```python
from build123d import *

# Parameters (mm, degrees)
SKETCH_1_W      = 33
SKETCH_1_H      = 18
EXTRUDE_1_DEPTH = 1.5
EXTRUDE_2_DEPTH = 0.6
EXTRUDE_3_DEPTH = 2


with BuildPart() as part:
    # Эскиз1 → Бобышка-Вытянуть1 (new body)
    with BuildSketch(Plane.XY):
        with Locations((16.5, 9)):
            Rectangle(SKETCH_1_W, SKETCH_1_H)
    extrude(amount=EXTRUDE_1_DEPTH)

    # Эскиз2 → Бобышка-Вытянуть2 (add)
    with BuildSketch(Plane.XY.offset(1.5)):
        Polygon((18, 12.535533906), (21.535533906, 9), (18, 5.464466094), (14.464466094, 9), align=None)
    extrude(amount=EXTRUDE_2_DEPTH)

    # Эскиз3 → Бобышка-Вытянуть3 (add)
    with BuildSketch(Plane.XY.offset(1.5)):
        with BuildLine():
            Line((6.886292912, 6), (6.886292912, 12))
            ThreePointArc((6.886292912, 12), (8.886292912, 14), (10.886292912, 12))
            Line((10.886292912, 12), (10.886292912, 6))
            ThreePointArc((10.886292912, 6), (8.886292912, 4), (6.886292912, 6))
        make_face()
    extrude(amount=EXTRUDE_3_DEPTH)


solid = part.part
```
For this review, take the finished solid that the model builds, in its own axes (mm). A direction names the side the tool comes from. Round coordinates to 2 decimals unless told otherwise and drop trailing zeros. Write each loop counter-clockwise with the first axis right and the second up, starting at its lowest first coordinate (ties: lowest second). Pieces come first, ordered by that corner, then holes. Notation, with made-up numbers: (-13, 70) - (16, 70) arc R24 ccw to (16, 98) - close; hole circle Ø7 at (23.5, 74). An arc over 180 degrees is marked (long way). Use CSV: the item, a comma, the result in double quotes.
1) Add section B-B on y = 10. Write out the cut boundary in (x, z).
Conclusion:
outline,"(0, 0) - (33, 0) - (33, 1.5) - (20.54, 1.5) - (20.54, 2.1) - (15.46, 2.1) - (15.46, 1.5) - (10.89, 1.5) - (10.89, 3.5) - (6.89, 3.5) - (6.89, 1.5) - (0, 1.5) - close"
2) For faces 1 (the flat face through (19.793, 7.257, 1.796)), 2 (the flat face through (16, 7, 1.5)), 3 (the flat face through (19.743, 10.793, 1.796)), list the 3-axis set-ups (+Z, -Z, +X, -X, +Y, -Y) from which the entire face can be reached by the end or side of a thin tool; tool diameter is ignored.
Conclusion:
face 1,"+Z, +X, -Y"
face 2,"+Z"
face 3,"+Z, +X, +Y"
3) Add section C-C on z = 2.75. Write out the cut boundary in (x, y).
Conclusion:
outline,"(6.89, 6) arc R2 ccw to (10.89, 6) - (10.89, 12) arc R2 ccw to (6.89, 12) - close"
4) Clearance check with flat-ended pins moving along their axes: pin 1 Ø1.5 at (x, z) = (7.5, 3) entering from +Y; pin 2 Ø1.5 at (x, z) = (3.5, 3) entering from +Y; pin 3 Ø1 at (x, y) = (28.5, 3.5) entering from +Z; pin 4 Ø2 at (x, y) = (16.5, 8) entering from +Z. State where each tip first meets the part, or that it passes through.
Conclusion:
pin 1,"stops at y = 13.9"
pin 2,"passes through"
pin 3,"stops at z = 1.5"
pin 4,"stops at z = 2.1"
5) Wall thickness on line 1 along Z through (x, y) = (4, 13); line 2 along X through (y, z) = (9.5, 2.35); line 3 along X through (y, z) = (6, 1.7): over which ranges is each line inside the solid? List them lowest first. Write a range as from..to.
Conclusion:
line 1,"z = 0..1.5"
line 2,"x = 6.89..10.89"
line 3,"x = 6.89..10.89, 17.46..18.54"
6) Add section A-A on x = 10. Write out the cut boundary in (y, z), and give its area (3 significant figures).
Conclusion:
outline,"(0, 0) - (18, 0) - (18, 1.5) - (13.66, 1.5) - (13.66, 3.5) - (4.34, 3.5) - (4.34, 1.5) - (0, 1.5) - close"
area,"45.6 mm^2"
7) The part is to be moulded in two halves that separate along X. For faces 4 (the flat face through (16.207, 10.743, 1.796)), 5 (the flat face through (6.886, 9, 2)), 6 (the flat face through (16, 0, 1)), say which applies: pulls with the +X half, pulls with the -X half, needs draft (parallel to the pull), parting line crosses it, or undercut.
Conclusion:
face 4,"undercut"
face 5,"pulls with the -X half"
face 6,"needs draft"
8) Add section D-D on x = 31. Write out the cut boundary in (y, z), and give its area (3 significant figures).
Conclusion:
outline,"(0, 0) - (18, 0) - (18, 1.5) - (0, 1.5) - close"
area,"27.0 mm^2"
